from build123d import *

# Parameters (mm, degrees)
F0_W      = 46.5
F0_H      = 150
F1_DEPTH  = 104.5
F2_W      = 42
F2_H      = 100
F3_DEPTH  = 147.75
F4_W      = 74.5
F4_H      = 50
F5_DEPTH  = 2.25
F6_R      = 1.5
F7_DEPTH  = 2.25
F8_R      = 1.5
F9_DEPTH  = 2.25
F10_W     = 10
F10_H     = 3
F11_DEPTH = 5
F12_W     = 10
F12_H     = 3
F13_DEPTH = 5
F14_W     = 28
F14_H     = 47
F15_DEPTH = 2.25
F16_W     = 23
F16_H     = 17
F17_DEPTH = 2.25


with BuildPart() as f1:
    # F0 (on Front) → F1 (new body)
    with BuildSketch(Plane.XZ):
        with Locations((-23.25, -75)):
            Rectangle(F0_W, F0_H)
    extrude(amount=F1_DEPTH)

    # F2 (on face) → F3 (cut, through all)
    with BuildSketch(Plane.XY):
        with Locations((-23.25, -52.25)):
            Rectangle(F2_W, F2_H)
    extrude(amount=-F3_DEPTH, mode=Mode.SUBTRACT)

    # F4 (on face) → F5 (cut)
    with BuildSketch(Plane.YZ):
        with Locations((-42.25, -25)):
            Rectangle(F4_W, F4_H)
    extrude(amount=-F5_DEPTH, mode=Mode.SUBTRACT)

    # F6 (on face) → F7 (cut)
    with BuildSketch(Plane(origin=(-46.5, 0, 0), x_dir=(0, -1, 0), z_dir=(-1, 0, 0))):
        with Locations((11.25, -10)):
            Circle(F6_R)
        with Locations((93.25, -10)):
            Circle(F6_R)
    extrude(amount=-F7_DEPTH, mode=Mode.SUBTRACT)

    # F8 (on face) → F9 (cut)
    with BuildSketch(Plane(origin=(0, 0, 0), x_dir=(-1, 0, 0), z_dir=(0, 1, 0))):
        with Locations((23.25, -48)):
            Circle(F8_R)
    extrude(amount=-F9_DEPTH, mode=Mode.SUBTRACT)

    # F10 (on face) → F11 (join)
    with BuildSketch(Plane.XZ.offset(2.25)):
        with Locations((-39.25, -73.5)):
            Rectangle(F10_W, F10_H)
        with Locations((-7.25, -73.5)):
            Rectangle(F10_W, F10_H)
    extrude(amount=F11_DEPTH)

    # F12 (on face) → F13 (join)
    with BuildSketch(Plane(origin=(0, -102.25, 0), x_dir=(-1, 0, 0), z_dir=(0, 1, 0))):
        with Locations((39.25, -73.5)):
            Rectangle(F12_W, F12_H)
    extrude(amount=F13_DEPTH)

    # F14 (on face) → F15 (cut)
    with BuildSketch(Plane.XZ.offset(104.5)):
        with Locations((-23.25, -117.25)):
            Rectangle(F14_W, F14_H)
    extrude(amount=-F15_DEPTH, mode=Mode.SUBTRACT)

    # F16 (on face) → F17 (cut)
    with BuildSketch(Plane(origin=(0, 0, 0), x_dir=(-1, 0, 0), z_dir=(0, 1, 0))):
        with Locations((20.75, -132.25)):
            Rectangle(F16_W, F16_H)
    extrude(amount=-F17_DEPTH, mode=Mode.SUBTRACT)


solid = f1.part
Here's how the part is built. I have some questions about the finished solid (model axes, mm). A direction names the side the tool comes from. Coordinates: 2 decimals unless noted, no trailing zeros. Write each loop counter-clockwise with the first axis right and the second up, starting at its lowest first coordinate (ties: lowest second). Pieces come first, ordered by that corner, then holes.
Item 1: I want a section at A-A on z = -126. Write out the boundary of the cut face in (x, y).
Item 2: If I drill on line 1 (Y direction, x = -16.5, z = -88); line 2 (X direction, y = -54, z = -105.5); line 3 (Z direction, x = -45, y = -93), over which ranges is the centre line in solid material (lowest first)?
Item 3: I want a section at B-B on x = -30.5. Write out the boundary of the cut face in (y, z).
Item 4: Will these pins go through, and if not, where does the flat tip stop? pin 1 (12 mm diameter, centred on x = -19.5, y = -58.5, fed in from +Z); pin 2 (2.5 mm diameter, centred on x = -1, y = -40, fed in from +Z).
Item 5: On a 3-axis mill with a long thin cutter (end or side, diameter ignored), from which of +Z, -Z, +X, -X, +Y, -Y can I reach the whole of each face in a straight line? I mean faces 1 (the flat face through (-39, -5, -75)), 2 (the flat face through (-39, -5, -72)), 3 (the cylindrical face through (-22.925, -1.109, -49.464)), 4 (the cylindrical face through (-45.391, -94.636, -10.575)), 5 (the cylindrical face through (-45.39, -10.06, -10.91)). Say none if no direction works.
Item 6: I want a section at D-D on z = -25.5. Write out the boundary of the cut face in (x, y).
Item 7: If we mould it in two halves opening along Y, with no side actions, what happens to faces 6 (the flat face through (-39, -100, -72)), 7 (the flat face through (-46.5, -52, -76))? For each: +Y half, -Y half, draft (parallel to the pull), parting line (faces both ways), or undercut.
Item 8: I want a section at C-C on y = -34. Write out the boundary of the cut face in (x, z).
Findings below:
1. outline: (-46.5, -104.5) - (-37.25, -104.5) - (-37.25, -102.25) - (-44.25, -102.25) - (-44.25, -2.25) - (-32.25, -2.25) - (-32.25, 0) - (-46.5, 0) - close; (-9.25, -104.5) - (0, -104.5) - (0, 0) - (-9.25, 0) - (-9.25, -2.25) - (-2.25, -2.25) - (-2.25, -102.25) - (-9.25, -102.25) - close
2. line 1: y = -104.5 to -102.25, -2.25 to 0
2. line 2: x = -46.5 to -44.25, -2.25 to 0
2. line 3: z = -150 to -11.48, -8.52 to 0
3. outline: (-104.5, -150) - (0, -150) - (0, -140.75) - (-2.25, -140.75) - (-2.25, -147.75) - (-102.25, -147.75) - (-102.25, -140.75) - (-104.5, -140.75) - close; (-104.5, -93.75) - (-102.25, -93.75) - (-102.25, 0) - (-104.5, 0) - close; (-2.25, -123.75) - (0, -123.75) - (0, 0) - (-2.25, 0) - close
4. pin 1: stops at z = -147.75
4. pin 2: stops at z = -50
5. face 1: none
5. face 2: +Z
5. face 3: +Y
5. face 4: -X
5. face 5: +X, -X
6. outline: (-46.5, -104.5) - (0, -104.5) - (0, -79.5) - (-2.25, -79.5) - (-2.25, -102.25) - (-44.25, -102.25) - (-44.25, -2.25) - (-2.25, -2.25) - (-2.25, -5) - (0, -5) - (0, 0) - (-46.5, 0) - close
7. face 6: undercut
7. face 7: draft
8. outline: (-46.5, -150) - (0, -150) - (0, -50) - (-2.25, -50) - (-2.25, -147.75) - (-44.25, -147.75) - (-44.25, 0) - (-46.5, 0) - close
